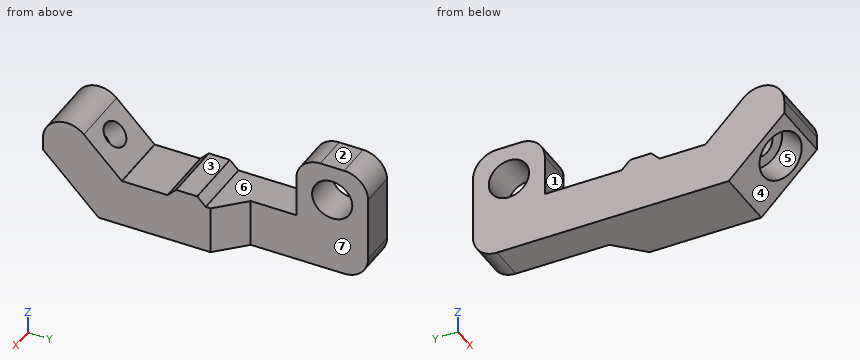
```python
from build123d import *

# Parameters (mm, degrees)
BOX013_W                    = 13
BOX013_H                    = 4.4
BOX013_DEPTH                = 1.8
CYLINDER007_R               = 5
CYLINDER007_DEPTH           = 6
CYLINDER007_PLACEMENT_ANGLE = 45
BOX011_W                    = 13
BOX011_H                    = 30
BOX011_DEPTH                = 50
BOX011_PLACEMENT_ANGLE      = 45
CYLINDER006_R               = 2.7
CYLINDER006_DEPTH           = 20
CYLINDER006_PLACEMENT_ANGLE = 45
BOX009_W                    = 13
BOX009_H                    = 10
BOX009_DEPTH                = 10
BOX008_W                    = 13
BOX008_H                    = 30
BOX008_DEPTH                = 50
BOX008_PLACEMENT_ANGLE      = 45
BOX007_W                    = 13
BOX007_H                    = 20
BOX007_DEPTH                = 30
CYLINDER005_R               = 4.2
CYLINDER005_DEPTH           = 10
BOX006_W                    = 7.5
BOX006_H                    = 15
BOX006_DEPTH                = 14
BOX005_W                    = 7.5
BOX005_H                    = 65
BOX005_DEPTH                = 10
BOX010_W                    = 5.5
BOX010_H                    = 35
BOX010_DEPTH                = 10
FILLET004_R                 = 5
CHAMFER001_SIZE             = 5.49
CHAMFER002_SIZE             = 1.79


with BuildPart() as cube009:
    # Box013 → Box013 (new body)
    with BuildSketch(Plane(origin=(0, 7.8, 0), x_dir=(1, 0, 0), z_dir=(0, 0, 1))):
        with Locations((6.5, 2.2)):
            Rectangle(BOX013_W, BOX013_H)
    extrude(amount=BOX013_DEPTH)


with BuildPart() as cylinder007:
    # Cylinder007 → Cylinder007 (new body)
    with BuildSketch(Plane.XY):
        Circle(CYLINDER007_R)
    extrude(amount=CYLINDER007_DEPTH)


with BuildPart() as cylinder007_1:
    # Cylinder007 placement: moved
    add(cylinder007.part.moved(Location((6.5, -15.970563, -2.727922))).rotate(Axis((6.5, -15.970563, -2.727922), (-1, 0, 0)), CYLINDER007_PLACEMENT_ANGLE))


with BuildPart() as box011:
    # Box011 → Box011 (new body)
    with BuildSketch(Plane.XY):
        with Locations((6.5, 15)):
            Rectangle(BOX011_W, BOX011_H)
    extrude(amount=BOX011_DEPTH)


with BuildPart() as box011_1:
    # Box011 placement: moved
    add(box011.part.moved(Location((0, -24.041631, -36.769553))).rotate(Axis((0, -24.041631, -36.769553), (1, 0, 0)), BOX011_PLACEMENT_ANGLE))


with BuildPart() as cylinder006:
    # Cylinder006 → Cylinder006 (new body)
    with BuildSketch(Plane.XY):
        Circle(CYLINDER006_R)
    extrude(amount=CYLINDER006_DEPTH)


with BuildPart() as cylinder006_1:
    # Cylinder006 placement: moved
    add(cylinder006.part.moved(Location((6.5, -22.334524, -9.091883))).rotate(Axis((6.5, -22.334524, -9.091883), (-1, 0, 0)), CYLINDER006_PLACEMENT_ANGLE))


with BuildPart() as cube008:
    # Box009 → Box009 (new body)
    with BuildSketch(Plane(origin=(0, -3.5, -0.5), x_dir=(1, 0, 0), z_dir=(0, 0, 1))):
        with Locations((6.5, 5)):
            Rectangle(BOX009_W, BOX009_H)
    extrude(amount=BOX009_DEPTH)


with BuildPart() as cube007:
    # Box008 → Box008 (new body)
    with BuildSketch(Plane.XY):
        with Locations((6.5, 15)):
            Rectangle(BOX008_W, BOX008_H)
    extrude(amount=BOX008_DEPTH)


with BuildPart() as cube007_1:
    # Box008 placement: moved
    add(cube007.part.moved(Location((0, -3.535534, 0))).rotate(Axis((0, -3.535534, 0), (1, 0, 0)), BOX008_PLACEMENT_ANGLE))


with BuildPart() as cut005:
    # Box007 → Box007 (new body)
    with BuildSketch(Plane(origin=(0, -20, -0.5), x_dir=(1, 0, 0), z_dir=(0, 0, 1))):
        with Locations((6.5, 10)):
            Rectangle(BOX007_W, BOX007_H)
    extrude(amount=BOX007_DEPTH)

    # Cut004: cut Cube007
    add(cube007_1.part, mode=Mode.SUBTRACT)

    # Cut005: cut Cube008-
    add(cube008.part, mode=Mode.SUBTRACT)


with BuildPart() as cylinder005:
    # Cylinder005 → Cylinder005 (new body)
    with BuildSketch(Plane(origin=(0, 37.5, 6), x_dir=(0, 0, -1), z_dir=(1, 0, 0))):
        Circle(CYLINDER005_R)
    extrude(amount=CYLINDER005_DEPTH)


with BuildPart() as cube005:
    # Box006 → Box006 (new body)
    with BuildSketch(Plane(origin=(0, 30, -0.5), x_dir=(1, 0, 0), z_dir=(0, 0, 1))):
        with Locations((3.75, 7.5)):
            Rectangle(BOX006_W, BOX006_H)
    extrude(amount=BOX006_DEPTH)


with BuildPart() as cut003:
    # Box005 → Box005 (new body)
    with BuildSketch(Plane(origin=(0, -20, -10), x_dir=(1, 0, 0), z_dir=(0, 0, 1))):
        with Locations((3.75, 32.5)):
            Rectangle(BOX005_W, BOX005_H)
    extrude(amount=BOX005_DEPTH)

    # Fusion003: union Cube005+
    add(cube005.part)

    # Cut003: cut Cylinder005-
    add(cylinder005.part, mode=Mode.SUBTRACT)


with BuildPart() as body001:
    # Box010 → Box010 (new body)
    with BuildSketch(Plane(origin=(7.5, -20, -10), x_dir=(1, 0, 0), z_dir=(0, 0, 1))):
        with Locations((2.75, 17.5)):
            Rectangle(BOX010_W, BOX010_H)
    extrude(amount=BOX010_DEPTH)

    # Fusion004: union Cut005, Cut003
    add(cut005.part)
    add(cut003.part)

    # Cut006: cut Cylinder006-
    add(cylinder006_1.part, mode=Mode.SUBTRACT)

    # Cut007: cut Box011
    add(box011_1.part, mode=Mode.SUBTRACT)

    # Cut009: cut Cylinder007
    add(cylinder007_1.part, mode=Mode.SUBTRACT)

    # Fusion005: union Cube009
    add(cube009.part)

    # Fillet004
    fillet004_edges = [body001.edges().sort_by_distance(p)[0] for p in [
        (3.75, 45, 13.5),
        (3.75, 30, 13.5),
        (6.5, -20, 16.464466),
        (3.75, 45, -10),
    ]]
    fillet(fillet004_edges, radius=FILLET004_R)

    # Chamfer001
    chamfer001_edges = [body001.edges().sort_by_distance(p)[0] for p in [
        (7.5, 15, -5),
    ]]
    chamfer(chamfer001_edges, length=CHAMFER001_SIZE)

    # Chamfer002
    chamfer002_edges = [body001.edges().sort_by_distance(p)[0] for p in [
        (10.25, 12.2, 0),
        (3.75, 12.2, 0),
        (3.75, 7.8, 0),
        (10.25, 7.8, 0),
    ]]
    chamfer(chamfer002_edges, length=CHAMFER002_SIZE)


solid = body001.part
```
Geometry check sheet. Reference: the model listing, model coordinates, mm. Face numbers are marked on the shaded views. A direction names the side the tool comes from. Coordinates: 2 decimals unless noted, no trailing zeros. Loops run counter-clockwise (first coordinate to the right, second up) from the corner with the lowest first, then second, coordinate; pieces in that order, holes last. Notation, with made-up numbers: (-9, -9) -> (29, -9) arc R29 cw to (29, 13) -> close; hole circle Ø5 at (56.25, 4). An arc over 180 degrees is marked (long way). Put each result on its own line as item: value.
1) Thickness scan on line 1 (Z direction, x = 2.25, y = 37.5); line 2 (Y direction, x = 1.75, z = 6); line 3 (Y direction, x = 1.25, z = 4.25). Record the ranges inside material, lowest first.
Result set:
line 1: z = -10 to 1.8, 10.2 to 13.5
line 2: y = -19.73 to -9.54, 30 to 33.3, 41.7 to 45
line 3: y = -20 to -7.79, 30 to 33.68, 41.32 to 45
2) Cross-section at A-A on y = 37.5. Record the boundary of the cut face in (x, z).
Result set:
outline: (0, -10) -> (7.5, -10) -> (7.5, 1.8) -> (0, 1.8) -> close; (0, 10.2) -> (7.5, 10.2) -> (7.5, 13.5) -> (0, 13.5) -> close
3) Gauge pin test, flat ends, axial feed: pin 1 Ø6.5 at (x, y) = (8.5, 21.5) entering from +Z; pin 2 Ø12 at (y, z) = (36, 3.5) entering from +X; pin 3 Ø7.5 at (y, z) = (37.5, 6) entering from -X; pin 4 Ø3 at (x, z) = (11, 0) entering from +Y. Record the tip position at first contact, or that the pin passes through.
Result set:
pin 1: stops at z = 0
pin 2: stops at x = 7.5
pin 3: passes through
pin 4: stops at y = 18.49
4) Tool access check on the marked faces 5, 6 and 7. Record the directions out of +Z, -Z, +X, -X, +Y, -Y that give a thin tool (end or side, any length) a straight path to the whole face; none if there is none.
Result set:
face 5: none
face 6: +Z, +X, -X
face 7: +Z, -Z, +X, +Y
5) Cross-section at C-C on y = 26. Record the boundary of the cut face in (x, z), plus the area to 3 significant figures.
Result set:
outline: (0, -10) -> (7.5, -10) -> (7.5, 0) -> (0, 0) -> close
area: 75.0 mm^2
6) Cross-section at B-B on x = 6. Count the separate pieces of the cut face and the enclosed holes in it, plus the area to 3 significant figures.
Result set:
separate pieces: 2
enclosed holes: 1
area: 747 mm^2
7) Release check for a two-part mould opening along Y. For the marked faces 1, 2, 3 and 4 record: released by +Y, released by -Y, zero draft, split by the parting line, or undercut.
Result set:
face 1: undercut
face 2: zero draft
face 3: undercut
face 4: released by -Y
